Check sheet for the modelled part. Datum: model origin and axes. Units: mm. Coordinates: 2 decimals unless noted, no trailing zeros. Answer as CSV lines item,"result". Start each with the question number.
1) Section check A-A (z = -1.25). State how many separate pieces and enclosed holes the cut face has, and give its area (3 significant figures).
2) Material ranges on L1, parallel to Y at x = 0, z = -0.55; L2, parallel to Y at x = 192.5, z = -1.3; L3, parallel to X at y = -44, z = -1.45, recorded low to high. Write a range as [from, to].
3) Go/stop test with flat-tipped pins: pin 1 Ø3.5 at (x, y) = (-174, -40) entering from +Z; pin 2 Ø1 at (x, z) = (-200, -1) entering from -Y; pin 3 Ø1 at (y, z) = (45.5, -1.5) entering from +X; pin 4 Ø1 at (y, z) = (-45, -1.5) entering from -X. Record where each tip stops, or that it passes through.
from build123d import *

# Parameters (mm, degrees)
BASE_FLANGE1_DEPTH    = 2
BREAK_CORNER1_START   = -2
BREAK_CORNER1_DEPTH   = 2
BREAK_CORNER1_2_DEPTH = 2
SKETCH2_R             = 2
CUT_EXTRUDE1_DEPTH    = 10
LPATTERN1_COUNT       = 3
LPATTERN1_PITCH       = 174


# Read off the part's stored shape, not the designer's step: Break-Corner1
# Sheet-metal steps are written as plain solids
with BuildPart() as part:
    # Sketch1 → Base-Flange1 (new body)
    with BuildSketch(Plane.XY):
        Polygon((189, -49), (-189, -49), (-189, -41), (-214, -41), (-214, 41), (-189, 41), (-189, 49), (189, 49), (189, 41), (214, 41), (214, -41), (189, -41), align=None)
    extrude(amount=-BASE_FLANGE1_DEPTH)

    # Break-Corner1 outline → Break-Corner1 (cut)
    with BuildSketch(Plane.XY.offset(BREAK_CORNER1_START)):
        with BuildLine():
            Line((214, 41), (211, 41))
            ThreePointArc((211, 41), (213.121320344, 40.121320344), (214, 38))
            Line((214, 38), (214, 41))
        make_face()
        with BuildLine():
            ThreePointArc((186, 49), (188.121320344, 48.121320344), (189, 46))
            Line((189, 46), (189, 49))
            Line((189, 49), (186, 49))
        make_face()
        with BuildLine():
            Line((214, -41), (214, -38))
            ThreePointArc((214, -38), (213.121320344, -40.121320344), (211, -41))
            Line((211, -41), (214, -41))
        make_face()
        with BuildLine():
            ThreePointArc((-189, 46), (-188.121320344, 48.121320344), (-186, 49))
            Line((-186, 49), (-189, 49))
            Line((-189, 49), (-189, 46))
        make_face()
        with BuildLine():
            Line((189, -49), (189, -46))
            ThreePointArc((189, -46), (188.121320344, -48.121320344), (186, -49))
            Line((186, -49), (189, -49))
        make_face()
        with BuildLine():
            ThreePointArc((-214, 38), (-213.121320344, 40.121320344), (-211, 41))
            Line((-211, 41), (-214, 41))
            Line((-214, 41), (-214, 38))
        make_face()
        with BuildLine():
            Line((-189, -49), (-186, -49))
            ThreePointArc((-186, -49), (-188.121320344, -48.121320344), (-189, -46))
            Line((-189, -46), (-189, -49))
        make_face()
        with BuildLine():
            ThreePointArc((-211, -41), (-213.121320344, -40.121320344), (-214, -38))
            Line((-214, -38), (-214, -41))
            Line((-214, -41), (-211, -41))
        make_face()
    extrude(amount=BREAK_CORNER1_DEPTH, mode=Mode.SUBTRACT)

    # Break-Corner1 2 outline → Break-Corner1 2 (add)
    with BuildSketch(Plane.XY.offset(BREAK_CORNER1_START)):
        with BuildLine():
            Line((189, 41), (192, 41))
            ThreePointArc((192, 41), (189.878679656, 41.878679656), (189, 44))
            Line((189, 44), (189, 41))
        make_face()
        with BuildLine():
            ThreePointArc((189, -44), (189.878679656, -41.878679656), (192, -41))
            Line((192, -41), (189, -41))
            Line((189, -41), (189, -44))
        make_face()
        with BuildLine():
            Line((-189, 41), (-189, 44))
            ThreePointArc((-189, 44), (-189.878679656, 41.878679656), (-192, 41))
            Line((-192, 41), (-189, 41))
        make_face()
        with BuildLine():
            ThreePointArc((-192, -41), (-189.878679656, -41.878679656), (-189, -44))
            Line((-189, -44), (-189, -41))
            Line((-189, -41), (-192, -41))
        make_face()
    extrude(amount=BREAK_CORNER1_2_DEPTH)

    # Sketch2 → Cut-Extrude1 (cut)
    with BuildSketch(Plane.XY):
        with Locations((-174, 40)):
            Circle(SKETCH2_R)
        with Locations((-174, -40)):
            Circle(SKETCH2_R)
    cut_extrude1 = extrude(amount=-CUT_EXTRUDE1_DEPTH, mode=Mode.SUBTRACT)

    # LPattern1: Cut-Extrude1 ×3
    with Locations(*[(i * LPATTERN1_PITCH, 0, 0) for i in range(1, LPATTERN1_COUNT)]):
        add(cut_extrude1, mode=Mode.SUBTRACT)


solid = part.part
Results found:
1,separate pieces,"1"
1,enclosed holes,"6"
1,area,"41,100 mm2"
2,L1,"y = [-49, -42], [-38, 38], [42, 49]"
2,L2,"y = [-41, 41]"
2,L3,"x = [-189, 189]"
3,pin 1,"passes through"
3,pin 2,"stops at y = -41"
3,pin 3,"stops at x = 189"
3,pin 4,"stops at x = -189"
